Verification items for this drawing (mm, ordinates from the low corner). Give positions to 0.01 mm unless a question says otherwise; leave off trailing zeros. Loops run counter-clockwise (first coordinate to the right, second up) from the corner with the lowest first, then second, coordinate; pieces in that order, holes last. Notation, with made-up numbers: (24.25, 68.25) -> (30.25, 68.25) arc R13 cw to (30.25, 82.25) -> close; hole circle Ø11 at (7, -3). An arc over 180 degrees is marked (long way). Write each question's results on one line, items separated by ' | '. Start each with the question number.
Item 1: Gauge pin test, flat end, axial feed: pin 1 Ø6 at (x, y) = (130.16, 24.21) entering from -Z. Record the tip position at first contact, or that the pin passes through.
Item 2: Cross-section at A-A on x = 30.16. Enter the section's corners in (y, z) (3 decimals).
Item 3: Cross-section at C-C on x = 10.16. Enter the section's corners in (y, z) (3 decimals).
Item 4: Scan lines: line 1 along Y through (x, z) = (30, 0.9); line 2 along Y through (x, z) = (130.5, 2.7); line 3 along Y through (x, z) = (95.16, 1.15). Record each from-to range of solid material in increasing order.
Item 5: Cross-section at B-B on y = 92.46. Enter the section's corners in (x, z) (3 decimals), then the cut area to 3 significant figures.
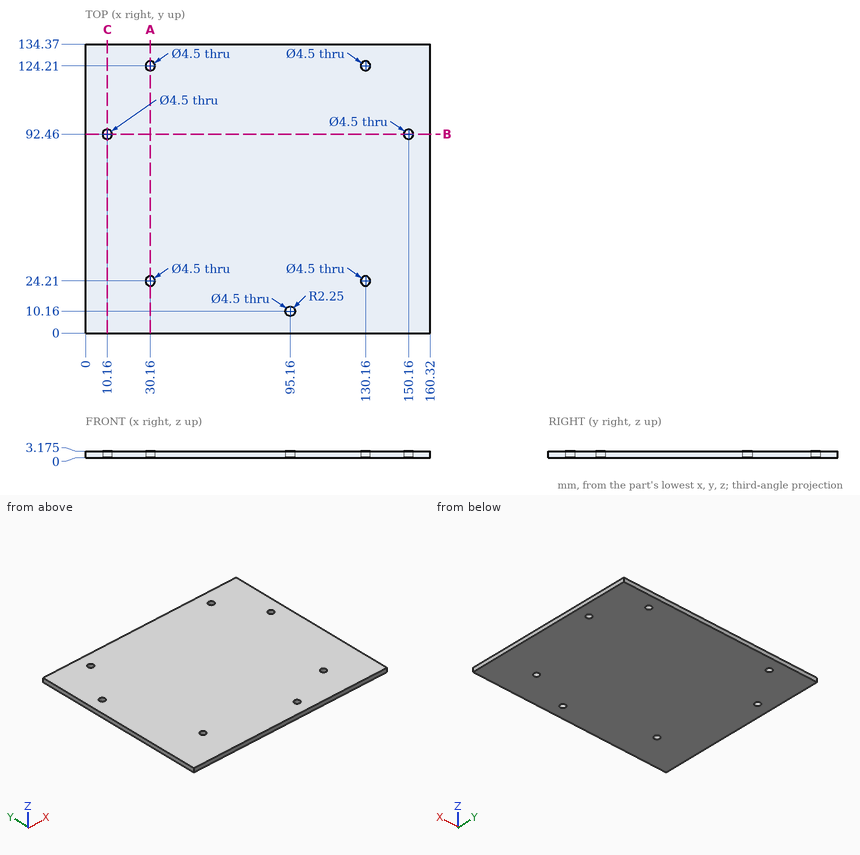
Answer sheet:
1) pin 1: stops at z = 0
2) outline: (0, 0) -> (21.96, 0) -> (21.96, 3.175) -> (0, 3.175) -> close; (26.46, 0) -> (121.96, 0) -> (121.96, 3.175) -> (26.46, 3.175) -> close; (126.46, 0) -> (134.37, 0) -> (134.37, 3.175) -> (126.46, 3.175) -> close
3) outline: (0, 0) -> (90.21, 0) -> (90.21, 3.175) -> (0, 3.175) -> close; (94.71, 0) -> (134.37, 0) -> (134.37, 3.175) -> (94.71, 3.175) -> close
4) line 1: y = 0 to 21.97, 26.45 to 121.97, 126.45 to 134.37 | line 2: y = 0 to 21.99, 26.43 to 121.99, 126.43 to 134.37 | line 3: y = 0 to 7.91, 12.41 to 134.37
5) outline: (0, 0) -> (7.91, 0) -> (7.91, 3.175) -> (0, 3.175) -> close; (12.41, 0) -> (147.91, 0) -> (147.91, 3.175) -> (12.41, 3.175) -> close; (152.41, 0) -> (160.32, 0) -> (160.32, 3.175) -> (152.41, 3.175) -> close | area: 480 mm²
